Check sheet for the modelled part. Datum: model origin and axes. Units: mm. Face numbers are marked on the shaded views. A direction names the side the tool comes from. Round coordinates to 2 decimals unless told otherwise and drop trailing zeros. Loops run counter-clockwise (first coordinate to the right, second up) from the corner with the lowest first, then second, coordinate; pieces in that order, holes last. Notation, with made-up numbers: (31.25, -26) -> (85.25, -26) arc R37 cw to (85.25, 13) -> close; hole circle Ø5 at (-17, 19.25). An arc over 180 degrees is marked (long way). Use one line per item in the form item = value. Start each with the question number.
(1) Sectioned sample at D-D (z = -1). Record the cut outline in (x, y), and give its area (3 significant figures).
(2) Sectioned sample at B-B (z = 38). Record the cut outline in (x, y), and give its area (3 significant figures).
(3) Set-up check for the marked faces 5 and 6: record each of +Z, -Z, +X, -X, +Y, -Y from which the full face is reachable in a straight line by a thin tool's end or side.
(4) Sectioned sample at A-A (y = -2.5). Record the cut outline in (x, z), and give its area (3 significant figures).
(5) Sectioned sample at C-C (y = 16). Record the cut outline in (x, z), and give its area (3 significant figures).
(6) Go/stop test with flat-tipped pins: pin 1 (11 mm diameter, centred on x = 25, z = -8, fed in from +Y); pin 2 (4 mm diameter, centred on x = -4, y = 18, fed in from +Z); pin 3 (2.5 mm diameter, centred on x = -53.5, z = 29, fed in from +Y). Record where each tip stops, or that it passes through.
(7) Material ranges on probe 1 along Z at (x, y) = (17.5, 31); probe 2 along Y at (x, z) = (-22, -9); probe 3 along Z at (x, y) = (-12, 3.5), recorded low to high. Write a range as [from, to].
(8) Draft check along X on the marked faces 1, 2, 3 and 4. Enter one of: released by +X, released by -X, zero draft, split by the parting line, or undercut.
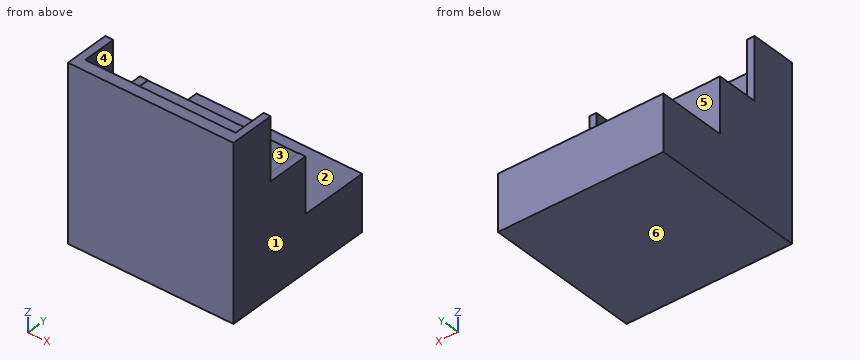
from build123d import *

# Parameters (mm, degrees)
F0_W          = 107.63935
F0_H          = 112.532053
F1_DEPTH      = 50.8
F1_DEPTH_BACK = 50.8
F2_W          = 107.63935
F2_H          = 76.294005
F3_DEPTH      = 44.704
F4_W          = 107.63935
F4_H          = 40.449448
F5_DEPTH      = 27.432
F7_W          = 97.853955
F7_H          = 88.931974
F8_DEPTH      = 41.656


with BuildPart() as f1:
    # F0 (on Front) → F1 (new body, two sides)
    with BuildSketch(Plane.XZ) as f1_sk:
        with Locations((-1.726836, 0.143902)):
            Rectangle(F0_W, F0_H)
    extrude(amount=F1_DEPTH)
    extrude(f1_sk.sketch, amount=-F1_DEPTH_BACK)

    # F2 (on face) → F3 (cut)
    with BuildSketch(Plane(origin=(0, 50.8, 0), x_dir=(-1, 0, 0), z_dir=(0, 1, 0))):
        with Locations((1.726836, 18.262926)):
            Rectangle(F2_W, F2_H)
    extrude(amount=-F3_DEPTH, mode=Mode.SUBTRACT)

    # F4 (on face) → F5 (cut)
    with BuildSketch(Plane(origin=(0, 6.096, 0), x_dir=(-1, 0, 0), z_dir=(0, 1, 0))):
        with Locations((1.726836, 36.185205)):
            Rectangle(F4_W, F4_H)
    extrude(amount=-F5_DEPTH, mode=Mode.SUBTRACT)

    # F7 (on offset) → F8 (cut)
    with BuildSketch(Plane.XY.offset(57.404)):
        with Locations((-1.43903, 1.00732)):
            Rectangle(F7_W, F7_H)
    extrude(amount=-F8_DEPTH, mode=Mode.SUBTRACT)


solid = f1.part
Checks:
q1.outline = (-55.55, -50.8) -> (52.09, -50.8) -> (52.09, 6.1) -> (-55.55, 6.1) -> close
q1.area = 6,120 mm2
q2.outline = (-55.55, -50.8) -> (52.09, -50.8) -> (52.09, -21.34) -> (47.49, -21.34) -> (47.49, -43.46) -> (-50.37, -43.46) -> (-50.37, -21.34) -> (-55.55, -21.34) -> close
q2.area = 1,010 mm2
q3.face_5 = +Z, +X, -X, +Y
q3.face_6 = -Z, +X, -X, +Y, -Y
q4.outline = (-55.55, -56.12) -> (52.09, -56.12) -> (52.09, 15.96) -> (47.49, 15.96) -> (47.49, 15.75) -> (-50.37, 15.75) -> (-50.37, 15.96) -> (-55.55, 15.96) -> close
q4.area = 7,740 mm2
q5.outline = (-55.55, -56.12) -> (52.09, -56.12) -> (52.09, -19.88) -> (-55.55, -19.88) -> close
q5.area = 3,900 mm2
q6.pin_1 = 6.1
q6.pin_2 = -19.88
q6.pin_3 = -21.34
q7.probe_1 = [-56.12, -19.88]
q7.probe_2 = [-50.8, 6.1]
q7.probe_3 = [-56.12, 15.75]
q8.face_1 = released by +X
q8.face_2 = zero draft
q8.face_3 = undercut
q8.face_4 = undercut
